```python
from build123d import *

# Parameters (mm, degrees)
SKETCH_R             = 27.5
PAD_DEPTH            = 1
SKETCH001_R          = 25.3
PAD001_DEPTH         = 6
SKETCH002_R          = 11
POCKET_DEPTH         = 6
SKETCH003_R          = 9.5
SKETCH003_R_2        = 14
POCKET001_DEPTH      = 7.001
POCKET001_DEPTH_BACK = -0.001
SKETCH004_R          = 1.45
POCKET002_DEPTH      = 27.501
POCKET002_DEPTH_BACK = -27.501
SKETCH005_R          = 1.45
POCKET003_DEPTH      = 27.501
POCKET003_DEPTH_BACK = -27.501


with BuildPart() as part:
    # Sketch → Pad (new body)
    with BuildSketch(Plane.XY):
        Circle(SKETCH_R)
    extrude(amount=PAD_DEPTH)

    # Sketch001 (on Face3 of Pad) → Pad001 (join)
    with BuildSketch(Plane.XY.offset(1)):
        Circle(SKETCH001_R)
    extrude(amount=PAD001_DEPTH)

    # Sketch002 (on Face5 of Pad001) → Pocket (cut)
    with BuildSketch(Plane.XY.offset(7)):
        Circle(SKETCH002_R)
    extrude(amount=-POCKET_DEPTH, mode=Mode.SUBTRACT)

    # Sketch003 (on Face5 of Pocket) → Pocket001 (cut, two sides)
    with BuildSketch(Plane.XY.offset(7)) as pocket001_sk:
        Circle(SKETCH003_R)
        with Locations((-19, 19)):
            Circle(SKETCH003_R_2)
        with Locations((19, 19)):
            Circle(SKETCH003_R_2)
        with Locations((-19, -19)):
            Circle(SKETCH003_R_2)
        with Locations((19, -19)):
            Circle(SKETCH003_R_2)
    extrude(amount=-POCKET001_DEPTH, mode=Mode.SUBTRACT)
    extrude(pocket001_sk.sketch, amount=-POCKET001_DEPTH_BACK, mode=Mode.SUBTRACT)

    # Sketch004 → Pocket002 (cut, two sides)
    with BuildSketch(Plane.XZ) as pocket002_sk:
        with Locations((0, 4)):
            Circle(SKETCH004_R)
    extrude(amount=-POCKET002_DEPTH, mode=Mode.SUBTRACT)
    extrude(pocket002_sk.sketch, amount=-POCKET002_DEPTH_BACK, mode=Mode.SUBTRACT)

    # Sketch005 → Pocket003 (cut, two sides)
    with BuildSketch(Plane.YZ) as pocket003_sk:
        with Locations((0, 4)):
            Circle(SKETCH005_R)
    extrude(amount=-POCKET003_DEPTH, mode=Mode.SUBTRACT)
    extrude(pocket003_sk.sketch, amount=-POCKET003_DEPTH_BACK, mode=Mode.SUBTRACT)


solid = part.part
```
Source: CAD feature listing. Evaluate the final solid. Frame: model axes, mm. A direction names the side the tool comes from. Round coordinates to 2 decimals unless told otherwise and drop trailing zeros. Write each loop counter-clockwise with the first axis right and the second up, starting at its lowest first coordinate (ties: lowest second). Pieces come first, ordered by that corner, then holes. Notation, with made-up numbers: M 72.25,68.5 L 117.25,68.5 A15 cw 117.25,77.5 Z; hole C -2,-2.75 d5. An arc over 180 degrees is marked long. Answer as a JSON object with one key per item and string values. Group by question number.
(1) Section query A-A on y = 0. Output: boundary loops of the cut face in (x, z), then the cut area to 3 significant figures.
(2) Ray query, line 1 (Z direction, x = 0, y = 15); line 2 (Z direction, x = -9.5, y = 2); line 3 (Y direction, x = 18.5, z = 2.25). Return the intervals inside material, ascending. Write a range as [from, to].
(3) Section query D-D on y = 19. Output: boundary loops of the cut face in (x, z), then the cut area to 3 significant figures.
(4) Mould query, pull axis X, two halves, no side actions, for faces 5 (the cylindrical face through (4.38, -8.43, 0.51)), 6 (the cylindrical face through (-25.258, 1.465, 3.291)), 7 (the flat face through (0, 26, 1)). Classes: +X half, -X half, draft (parallel to the pull), parting line (faces both ways), or undercut.
(5) Reachability of faces 1 (the cylindrical face through (1.465, 25.258, 3.291)), 2 (the flat face through (-10, 0, 1)), 3 (the cylindrical face through (25.258, -1.465, 3.291)), 4 (the cylindrical face through (-1.465, -25.258, 3.291)) from +Z, -Z, +X, -X, +Y, -Y: full face, straight path, thin tool, end or side. Return the list, or none.
(6) Section query C-C on z = 6.25. Output: boundary loops of the cut face in (x, y), then the cut area to 3 significant figures.
(7) First-contact query: pin 1 (2.5 mm diameter, centred on x = 0, z = 4, fed in from +Y); pin 2 (0.9 mm diameter, centred on x = 26, y = 2, fed in from +Z); pin 3 (4 mm diameter, centred on x = 0, z = 4, fed in from -Y); pin 4 (3 mm diameter, centred on y = 3.5, z = 1.5, fed in from +X). Flat tips, straight axial feed; report the tip coordinate or a pass-through.
Computed values:
{
 "1": {"outline": "M -27.5,0 L -9.5,0 L -9.5,1 L -11,1 L -11,2.55 L -25.3,2.55 L -25.3,1 L -27.5,1 Z; M -25.3,5.45 L -11,5.45 L -11,7 L -25.3,7 Z; M 9.5,0 L 27.5,0 L 27.5,1 L 25.3,1 L 25.3,2.55 L 11,2.55 L 11,1 L 9.5,1 Z; M 11,5.45 L 25.3,5.45 L 25.3,7 L 11,7 Z", "area": "125 mm^2"},
 "2": {"line 1": "[0, 2.55], [5.45, 7]", "line 2": "[0, 1]", "line 3": "[-5.01, 5.01]"},
 "3": {"outline": "M -5,0 L 5,0 L 5,7 L -5,7 Z; hole C 0,4 d2.9", "area": "63.4 mm^2"},
 "4": {"face 5": "undercut", "face 6": "-X half", "face 7": "draft"},
 "5": {"face 1": "+Z, +Y", "face 2": "+Z", "face 3": "+Z, +X", "face 4": "+Z, -Y"},
 "6": {"outline": "M -24.54,-6.14 A14 cw -6.14,-24.54 A25.3 ccw 6.14,-24.54 A14 cw 24.54,-6.14 A25.3 ccw 24.54,6.14 A14 cw 6.14,24.54 A25.3 ccw -6.14,24.54 A14 cw -24.54,6.14 A25.3 ccw Z; hole C 0,0 d22", "area": "711 mm^2"},
 "7": {"pin 1": "through", "pin 2": "z = 1", "pin 3": "y = -25.3", "pin 4": "x = 27.42"}
}
